Geometry check sheet. Reference: the model listing, model coordinates, mm. A direction names the side the tool comes from. Round coordinates to 2 decimals unless told otherwise and drop trailing zeros. Loops run counter-clockwise (first coordinate to the right, second up) from the corner with the lowest first, then second, coordinate; pieces in that order, holes last. Notation, with made-up numbers: M 39,3.5 L 56,3.5 A30 cw 56,37.5 Z; hole C -24,-27.75 d6. An arc over 180 degrees is marked long. Use one line per item in the form item = value. Start each with the question number.
1. Material ranges on line 1 (Y direction, x = 0, z = 2.2); line 2 (Y direction, x = 0, z = 64.95); line 3 (Z direction, x = -1.5, y = 6), recorded low to high.
2. Draft check along X on faces 4 (the cylindrical face through (4, 0, 2)), 5 (the flat face through (0, 0, 0)), 6 (the cylindrical face through (-1.172, 8.923, 32.045)). Enter one of: pulls with the +X half, pulls with the -X half, needs draft (parallel to the pull), parting line crosses it, or undercut.
3. Cross-section at C-C (z = 29.5). Record the boundary of the cut face in (x, y), then the cut area to 3 significant figures.
4. Cross-section at A-A (x = 0). Record the boundary of the cut face in (y, z), then the cut area to 3 significant figures.
5. Go/stop test with flat-tipped pins: pin 1 (1 mm diameter, centred on y = -6, z = 21, fed in from +X); pin 2 (7 mm diameter, centred on x = -1.5, y = -3, fed in from +Z); pin 3 (6 mm diameter, centred on x = -4, z = 34, fed in from +Y). Record where each tip stops, or that it passes through.
6. Cross-section at D-D (y = 7.75). Record the boundary of the cut face in (x, z).
7. Set-up check for faces 1 (the flat face through (2, -6, 0)), 2 (the flat face through (0, 0, 64.8)), 3 (the cylindrical face through (-3.865, -3.913, 2.57)): record each of +Z, -Z, +X, -X, +Y, -Y from which the full face is reachable in a straight line by a thin tool's end or side.
```python
from build123d import *

# Parameters (mm, degrees)
CYLINDER_R      = 9
CYLINDER_DEPTH  = 65
SKETCH_R        = 7
POCKET_DEPTH    = 0.2
SKETCH001_R     = 6
POCKET001_DEPTH = 4
PAD_DEPTH       = 4
FILLET_R        = 1.1


with BuildPart() as part:
    # Cylinder → Cylinder (new body)
    with BuildSketch(Plane.XY):
        Circle(CYLINDER_R)
    extrude(amount=CYLINDER_DEPTH)

    # Sketch (on Face3 of BaseFeature) → Pocket (cut)
    with BuildSketch(Plane.XY.offset(65)):
        Circle(SKETCH_R)
    extrude(amount=-POCKET_DEPTH, mode=Mode.SUBTRACT)

    # Sketch001 (on Face2 of Pocket) → Pocket001 (cut)
    with BuildSketch(Plane(origin=(0, 0, 0), x_dir=(1, 0, 0), z_dir=(0, 0, -1))):
        Circle(SKETCH001_R)
    extrude(amount=-POCKET001_DEPTH, mode=Mode.SUBTRACT)

    # Sketch002 (on Face6 of Pocket001) → Pad (join)
    with BuildSketch(Plane(origin=(0, 0, 4), x_dir=(1, 0, 0), z_dir=(0, 0, -1))):
        with BuildLine():
            ThreePointArc((-5.1875, -1.827524), (-3.889087, -3.889087), (-1.827524, -5.1875))
            ThreePointArc((1.827524, -5.1875), (0, -4), (-1.827524, -5.1875))
            ThreePointArc((1.827524, -5.1875), (3.889087, -3.889087), (5.1875, -1.827524))
            ThreePointArc((5.1875, 1.827524), (4, 0), (5.1875, -1.827524))
            ThreePointArc((5.1875, 1.827524), (3.889087, 3.889087), (1.827524, 5.1875))
            ThreePointArc((-1.827524, 5.1875), (0, 4), (1.827524, 5.1875))
            ThreePointArc((-1.827524, 5.1875), (-3.889087, 3.889087), (-5.1875, 1.827524))
            ThreePointArc((-5.1875, -1.827524), (-4, 0), (-5.1875, 1.827524))
        make_face()
    extrude(amount=PAD_DEPTH)

    # Fillet
    fillet_edges = [part.edges().sort_by_distance(p)[0] for p in [
        (-3.889087, 3.889087, 0),
        (3.889087, 3.889087, 0),
        (3.889087, -3.889087, 0),
        (-3.889087, -3.889087, 0),
    ]]
    fillet(fillet_edges, radius=FILLET_R)


solid = part.part
```
Reported:
q1.line_1 = -9 to -6, -4 to 4, 6 to 9
q1.line_2 = -9 to -7, 7 to 9
q1.line_3 = 0 to 64.8
q2.face_4 = undercut
q2.face_5 = needs draft
q2.face_6 = parting line crosses it
q3.outline = C 0,0 d18
q3.area = 254 mm²
q4.outline = M -9,0 L -6,0 L -6,4 L -4,4 L -4,0 L 4,0 L 4,4 L 6,4 L 6,0 L 9,0 L 9,65 L 7,65 L 7,64.8 L -7,64.8 L -7,65 L -9,65 Z
q4.area = 1,150 mm²
q5.pin_1 = 7.12
q5.pin_2 = 64.8
q5.pin_3 = 8.94
q6.outline = M -4.58,0 L 4.58,0 L 4.58,65 L -4.58,65 Z
q7.face_1 = -Z, +X, -X, +Y, -Y
q7.face_2 = +Z
q7.face_3 = -Z
